Input: part model. Units: mm. Frame: model coordinates. A direction names the side the tool comes from. Give positions to 0.01 mm unless a question says otherwise; leave off trailing zeros. Order: outer loops, then holes, each group sorted by start corner. A loop starts at its lowest first (then second) coordinate and runs counter-clockwise, first axis right, second up. Notation, with made-up numbers: (-21.75, 4.5) - (-3.75, 4.5) arc R20 cw to (-3.75, 25.5) - close; hole circle Ø6 at (48, -9). An arc over 180 degrees is marked (long way). Use a Markdown table: item, result.
from build123d import *

# Parameters (mm, degrees)
BOSS_EXTRUDE5_DEPTH = 15
BOSS_EXTRUDE6_DEPTH = 2
FILLET2_R           = 1.5
SKETCH7_W           = 13.5
SKETCH7_H           = 12
CUT_EXTRUDE2_DEPTH  = 5
FILLET3_R           = 6.2


with BuildPart() as part:
    # Sketch4 → Boss-Extrude5 (new body)
    with BuildSketch(Plane(origin=(0, 0, 0), x_dir=(1, 0, 0), z_dir=(0, 1, 0))):
        with BuildLine():
            Line((-60, -3), (-94.871191548, -3))
            ThreePointArc((-94.871191548, -3), (-83.664319132, -25.787593916), (-60, -35))
            Line((-60, -35), (-60, -3))
        make_face()
        with BuildLine():
            Line((-62, -5), (-93.12476415, -5))
            ThreePointArc((-93.12476415, -5), (-82.597547458, -24.730565074), (-62, -33.440245214))
            Line((-62, -33.440245214), (-62, -5))
        make_face(mode=Mode.SUBTRACT)
    extrude(amount=BOSS_EXTRUDE5_DEPTH)

    # Sketch5 → Boss-Extrude6 (add)
    with BuildSketch(Plane(origin=(0, 15, 0), x_dir=(1, 0, 0), z_dir=(0, 1, 0))):
        with BuildLine():
            Line((-60, -3), (-94.871191548, -3))
            ThreePointArc((-94.871191548, -3), (-83.664319132, -25.787593916), (-60, -35))
            Line((-60, -35), (-60, -3))
        make_face()
    extrude(amount=BOSS_EXTRUDE6_DEPTH)

    # Fillet2
    fillet2_edges = [part.edges().sort_by_distance(p)[0] for p in [
        (-60, 17, 19),
        (-77.435595774, 17, 3),
        (-83.664319132, 17, 25.787593916),
    ]]
    fillet(fillet2_edges, radius=FILLET2_R)

    # Sketch7 → Cut-Extrude2 (cut)
    with BuildSketch(Plane(origin=(-60, 0, 0), x_dir=(0, 0, -1), z_dir=(1, 0, 0))):
        with Locations((-13.25, 6)):
            Rectangle(SKETCH7_W, SKETCH7_H)
    extrude(amount=-CUT_EXTRUDE2_DEPTH, mode=Mode.SUBTRACT)

    # Fillet3
    fillet3_edges = [part.edges().sort_by_distance(p)[0] for p in [
        (-61, 12, 20),
        (-61, 12, 6.5),
    ]]
    fillet(fillet3_edges, radius=FILLET3_R)


solid = part.part
1. Set-up query: faces 4 (the face through (-77.68, 16.55, 3.43)), 5 (the face through (-61, 12, 13)), 6 (the face through (-77, 7, 5)). Return all of +Z, -Z, +X, -X, +Y, -Y with unobstructed straight access to the full face (end or side cutting, diameter ignored); none if empty.
Response:
| item | result |
|---|---|
| face 4 | -Z, +X, -X, +Y |
| face 5 | +X, -Y |
| face 6 | -Y |
2. Material intervals for line 1 along X through (y, z) = (14.25, 30); line 2 along Y through (x, z) = (-86.5, 20); line 3 along X through (y, z) = (11.75, 9), sorted ascending.
Response:
| item | result |
|---|---|
| line 1 | x = -78.03 to -74.91, -62 to -60 |
| line 2 | y = 15 to 17 |
| line 3 | x = -93.82 to -92.27, -62 to -60 |
3. Pin query (flat end, axial travel): pin 1 (7.5 mm diameter, centred on x = -78, y = 8, fed in from +Z); pin 2 (1 mm diameter, centred on y = 9, z = 19, fed in from -X); pin 3 (2 mm diameter, centred on x = -77.5, y = 4.5, fed in from +Z). Return the tip coordinate at first contact, or that it passes through.
Response:
| item | result |
|---|---|
| pin 1 | stops at z = 31.97 |
| pin 2 | stops at x = -89.71 |
| pin 3 | stops at z = 30.87 |
4. Section query C-C (y = 11.25). Return loops of the section in (x, z), then the cut area to 3 significant figures.
Response:
| item | result |
|---|---|
| outline | (-94.87, 3) - (-60, 3) - (-60, 9.74) - (-62, 9.74) - (-62, 5) - (-93.12, 5) arc R33.5 cw to (-62, 33.44) - (-62, 16.76) - (-60, 16.76) - (-60, 35) arc R35 ccw to start |
| area | 186 mm^2 |
5. Mould query, pull axis X, two halves, no side actions, for faces 1 (the face through (-82.832, 7.395, 24.514)), 2 (the face through (-60.45, 16.57, 18.78)), 3 (the face through (-61, 3, 6.5)). Classes: pulls with the +X half, pulls with the -X half, needs draft (parallel to the pull), parting line crosses it, or undercut.
Response:
| item | result |
|---|---|
| face 1 | undercut |
| face 2 | pulls with the +X half |
| face 3 | needs draft |
6. Section query B-B (y = 6.75). Return loops of the section in (x, z), then the cut area to 3 significant figures.
Response:
| item | result |
|---|---|
| outline | (-94.87, 3) - (-60, 3) - (-60, 6.57) - (-62, 6.57) - (-62, 5) - (-93.12, 5) arc R33.5 cw to (-62, 33.44) - (-62, 19.93) - (-60, 19.93) - (-60, 35) arc R35 ccw to start |
| area | 173 mm^2 |
7. Section query A-A (y = 13.5). Return loops of the section in (x, z), then the cut area to 3 significant figures.
Response:
| item | result |
|---|---|
| outline | (-94.87, 3) - (-60, 3) - (-60, 35) arc R35 ccw to start; hole (-93.12, 5) - (-62, 5) - (-62, 33.44) arc R33.5 ccw to start |
| area | 200 mm^2 |
